```python
from build123d import *

# Parameters (mm, degrees)
F0_R     = 25.4
F1_DEPTH = 3.429


with BuildPart() as f1:
    # F0 (on Front) → F1 (new body)
    with BuildSketch(Plane.XZ):
        Polygon((205.224228, -4.022674), (205.224228, -7.197674), (186.174228, -7.197674), (186.174228, -4.022674), (-15.755772, -4.022674), (-15.755772, -7.197674), (-34.805772, -7.197674), (-34.805772, -4.022674), (-105.290772, -4.022674), (-105.290772, -45.932674), (-108.465772, -45.932674), (-108.465772, -63.712674), (-105.290772, -63.712674), (-105.290772, -105.622674), (55.046728, -105.622674), (55.046728, -87.461674), (115.371728, -87.461674), (115.371728, -105.622674), (275.709228, -105.622674), (275.709228, -63.712674), (278.884228, -63.712674), (278.884228, -45.932674), (275.709228, -45.932674), (275.709228, -4.022674), align=None)
        with Locations((84.713775, -54.844671)):
            Circle(F0_R, mode=Mode.SUBTRACT)
        with Locations((-54.350514, -54.822674)):
            Circle(F0_R, mode=Mode.SUBTRACT)
        with Locations((15.486786, -54.822674)):
            Circle(F0_R, mode=Mode.SUBTRACT)
        with Locations((154.931694, -54.822674)):
            Circle(F0_R, mode=Mode.SUBTRACT)
        with Locations((224.768994, -54.822674)):
            Circle(F0_R, mode=Mode.SUBTRACT)
    extrude(amount=F1_DEPTH)


solid = f1.part
```
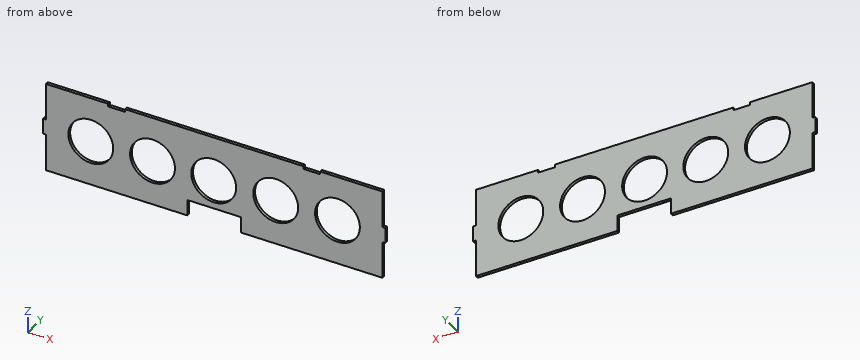
CAD build for the part. Positions are in the model's coordinates, mm. Coordinates: 2 decimals unless noted, no trailing zeros. Write each loop counter-clockwise with the first axis right and the second up, starting at its lowest first coordinate (ties: lowest second). Pieces come first, ordered by that corner, then holes. Notation, with made-up numbers: (41.5, 30.5) -> (67.5, 30.5) arc R30 ccw to (67.5, 68.5) -> close; hole circle Ø5 at (84.25, 14). An arc over 180 degrees is marked (long way). Return JSON: item names as keys, results as strings. Group by question number.
Q1. Cut at A-A, the plane z = -73.5. Give the cut face in (x, y).
Q2. Drill centre lines: line 1 (X direction, y = -1.35, z = -99.5); line 2 (X direction, y = -2.3, z = -57); line 3 (X direction, y = -3.05, z = -60.5). Where is each one in solid material? Low to high.
Q3. Cut at C-C, the plane y = -2.3. State how many separate pieces and enclosed holes the cut face has, then the cut area to 3 significant figures.
Q4. Cut at D-D, the plane x = 101.5. Give the cut face in (y, z).
Q5. Cut at B-B, the plane x = 19. Give the cut face in (y, z).
Q6. Flat gauge pins, fed straight in: pin 1 (1 mm diameter, centred on y = -1.5, z = -6, fed in from -X); pin 2 (1.7 mm diameter, centred on y = -1, z = -77, fed in from +X); pin 3 (1 mm diameter, centred on x = 194, y = -2.5, fed in from +Z). Where does each tip first touch, or does it go through?
Returned:
{
 "1": {"outline": "(-105.29, -3.43) -> (-71.56, -3.43) -> (-71.56, 0) -> (-105.29, 0) -> close; (-37.14, -3.43) -> (-1.73, -3.43) -> (-1.73, 0) -> (-37.14, 0) -> close; (32.7, -3.43) -> (67.48, -3.43) -> (67.48, 0) -> (32.7, 0) -> close; (101.95, -3.43) -> (137.72, -3.43) -> (137.72, 0) -> (101.95, 0) -> close; (172.15, -3.43) -> (207.56, -3.43) -> (207.56, 0) -> (172.15, 0) -> close; (241.98, -3.43) -> (275.71, -3.43) -> (275.71, 0) -> (241.98, 0) -> close"},
 "2": {"line 1": "x = -105.29 to 55.05, 115.37 to 275.71", "line 2": "x = -108.47 to -79.66, -29.04 to -9.82, 40.79 to 59.41, 110.02 to 129.63, 180.24 to 199.46, 250.08 to 278.88", "line 3": "x = -108.47 to -79.11, -29.59 to -9.27, 40.24 to 59.95, 109.48 to 130.17, 179.69 to 200.01, 249.53 to 278.88"},
 "3": {"separate pieces": "1", "enclosed holes": "5", "area": "27,500 mm2"},
 "4": {"outline": "(-3.43, -87.46) -> (0, -87.46) -> (0, -73.91) -> (-3.43, -73.91) -> close; (-3.43, -35.78) -> (0, -35.78) -> (0, -4.02) -> (-3.43, -4.02) -> close"},
 "5": {"outline": "(-3.43, -105.62) -> (0, -105.62) -> (0, -79.98) -> (-3.43, -79.98) -> close; (-3.43, -29.67) -> (0, -29.67) -> (0, -4.02) -> (-3.43, -4.02) -> close"},
 "6": {"pin 1": "stops at x = -105.29", "pin 2": "stops at x = 275.71", "pin 3": "stops at z = -7.2"}
}
